Design review of the part built by this model. Coordinates are the model's own, in mm. A direction names the side the tool comes from. Coordinates: 2 decimals unless noted, no trailing zeros. Loops run counter-clockwise (first coordinate to the right, second up) from the corner with the lowest first, then second, coordinate; pieces in that order, holes last. Notation, with made-up numbers: (79, -20) - (115, -20) arc R10 cw to (115, -4) - close; hole circle Ø1 at (-20, 25.5). An arc over 180 degrees is marked (long way). Answer in a Markdown table with one row per item. Add a question column.
(1) Clearance check with flat-ended pins moving along their axes: pin 1 (1 mm diameter, centred on x = -0.5, y = -26, fed in from +Z); pin 2 (1.5 mm diameter, centred on x = -3, y = -1.5, fed in from -Z); pin 3 (6 mm diameter, centred on y = -15, z = 1.5, fed in from +X). State where each tip first meets the part, or that it passes through.
(2) We need section D-D, the plane y = -31. Write out the cut boundary in (x, z), plus the area to 3 significant figures.
(3) To check wall thickness, follow L1, parallel to Y at x = 7, z = -5; L2, parallel to X at y = 2.5, z = -2.5; L3, parallel to Z at x = -0.25, y = -26.5. State the ranges of each line that lie inside material, in increasing order. Write a range as [from, to].
(4) For faces 1 (the face through (-2.38, -3.94, -10.74)), 2 (the face through (-11.99, 1.97, -0.53)), list the 3-axis set-ups (+Z, -Z, +X, -X, +Y, -Y) from which the entire face can be reached by the end or side of a thin tool; tool diameter is ignored.
(5) We need section A-A, the plane z = 0. Write out the cut boundary in (x, y).
(6) We need section C-C, the plane y = -17. Write out the cut boundary in (x, z), plus the area to 3 significant figures.
(7) We need section B-B, the plane x = 0. Write out the cut boundary in (y, z), plus the area to 3 significant figures.
from build123d import *

# Parameters (mm, degrees)
ESQUISSE1_R      = 12
EXTRUSION1_DEPTH = 7
ESQUISSE2_R      = 11
EXTRUSION2_DEPTH = 8
CONG_1_R         = 3
ESQUISSE3_R      = 10
EXTRUSION3_DEPTH = 5
ESQUISSE4_R      = 9
EXTRUSION4_DEPTH = 7
ESQUISSE5_R      = 7.5
EXTRUSION5_DEPTH = 15


with BuildPart() as part:
    # Esquisse1 → Extrusion1 (new body)
    with BuildSketch(Plane(origin=(0, 0, 0), x_dir=(1, 0, 0), z_dir=(0, 1, 0))):
        Circle(ESQUISSE1_R)
    extrude(amount=EXTRUSION1_DEPTH)

    # Esquisse2 → Extrusion2 (add)
    with BuildSketch(Plane.XZ):
        Circle(ESQUISSE2_R)
    extrude(amount=EXTRUSION2_DEPTH)

    # Congé1
    cong_1_edges = [part.edges().sort_by_distance(p)[0] for p in [
        (-12, 7, 0),
    ]]
    fillet(cong_1_edges, radius=CONG_1_R)

    # Esquisse3 → Extrusion3 (add)
    with BuildSketch(Plane.XZ.offset(8)):
        Circle(ESQUISSE3_R)
    extrude(amount=EXTRUSION3_DEPTH)

    # Esquisse4 → Extrusion4 (add)
    with BuildSketch(Plane.XZ.offset(13)):
        Circle(ESQUISSE4_R)
    extrude(amount=EXTRUSION4_DEPTH)

    # Esquisse5 → Extrusion5 (add)
    with BuildSketch(Plane.XZ.offset(20)):
        Circle(ESQUISSE5_R)
    extrude(amount=EXTRUSION5_DEPTH)


solid = part.part
Responses:
| question | item | result |
|---|---|---|
| 1 | pin 1 | stops at z = 7.5 |
| 1 | pin 2 | stops at z = -10.77 |
| 1 | pin 3 | stops at x = 10 |
| 2 | outline | circle Ø15 at (0, 0) |
| 2 | area | 177 mm2 |
| 3 | L1 | y = [-20, 7] |
| 3 | L2 | x = [-11.74, 11.74] |
| 3 | L3 | z = [-7.5, 7.5] |
| 4 | face 1 | -Y |
| 4 | face 2 | +Y, -Y |
| 5 | outline | (-12, 0) - (-11, 0) - (-11, -8) - (-10, -8) - (-10, -13) - (-9, -13) - (-9, -20) - (-7.5, -20) - (-7.5, -35) - (7.5, -35) - (7.5, -20) - (9, -20) - (9, -13) - (10, -13) - (10, -8) - (11, -8) - (11, 0) - (12, 0) - (12, 4) arc R3 ccw to (9, 7) - (-9, 7) arc R3 ccw to (-12, 4) - close |
| 6 | outline | circle Ø18 at (0, 0) |
| 6 | area | 254 mm2 |
| 7 | outline | (-35, -7.5) - (-20, -7.5) - (-20, -9) - (-13, -9) - (-13, -10) - (-8, -10) - (-8, -11) - (0, -11) - (0, -12) - (4, -12) arc R3 ccw to (7, -9) - (7, 9) arc R3 ccw to (4, 12) - (0, 12) - (0, 11) - (-8, 11) - (-8, 10) - (-13, 10) - (-13, 9) - (-20, 9) - (-20, 7.5) - (-35, 7.5) - close |
| 7 | area | 791 mm2 |
